Part print with two shaded views. Sizes in mm from the minimum x, y, z corner. Give positions to 0.01 mm unless a question says otherwise; leave off trailing zeros. Write each loop counter-clockwise with the first axis right and the second up, starting at its lowest first coordinate (ties: lowest second). Pieces come first, ordered by that corner, then holes.
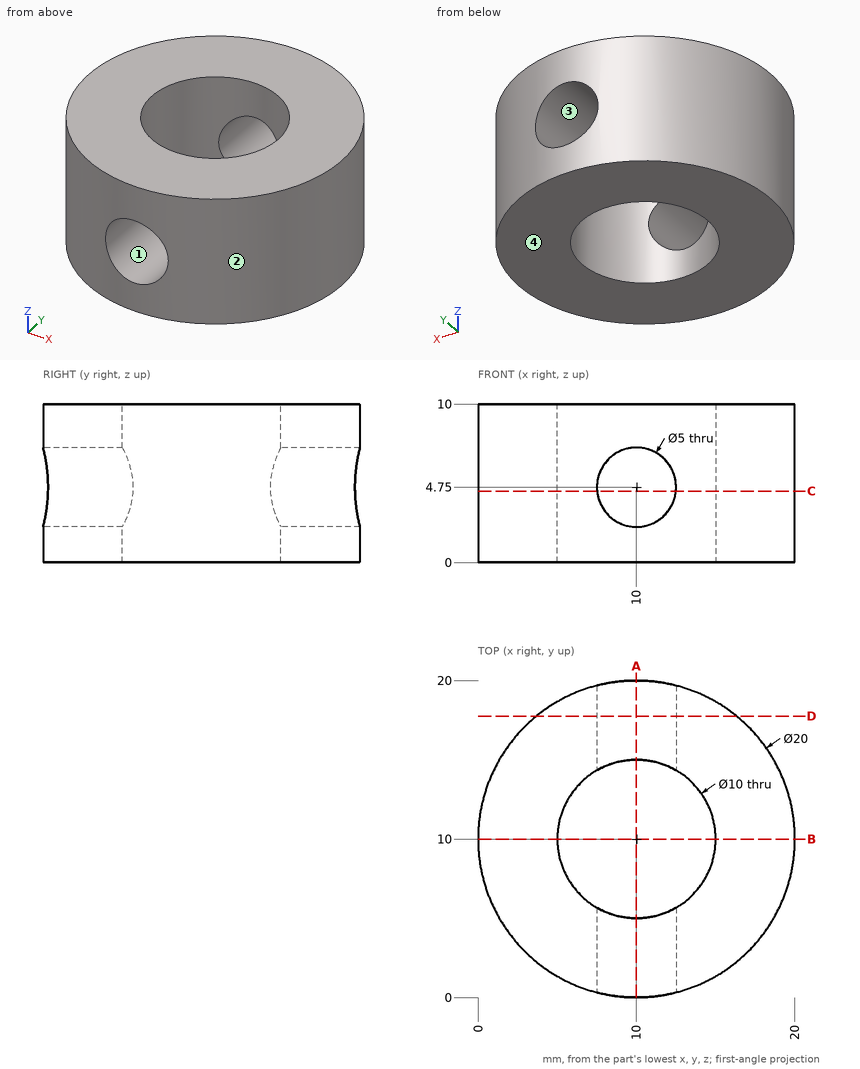
1) Flat gauge pins, fed straight in: P1, Ø2, axis at x = 7.5, z = 8.5, coming from the +Y side; P2, Ø2, axis at x = 14, z = 2, coming from the +Y side; P3, Ø1, axis at x = 3, z = 6.5, coming from the -Y side. Where does each tip first touch, or does it go through?
Check result:
P1: stops at y = 19.89
P2: stops at y = 19.54
P3: stops at y = 2.4
2) Saw through at D-D (y = 17.75). Write the cut outline in (x, z), and give its area (3 significant figures).
Check result:
outline: (3.68, 0) - (16.32, 0) - (16.32, 10) - (3.68, 10) - close; hole circle Ø5 at (10, 4.75)
area: 107 mm2
3) Saw through at C-C (z = 4.5). Write the cut outline in (x, y), and give its area (3 significant figures).
Check result:
outline: (7.51, 0.31) - (7.51, 5.66) arc R5 cw to (7.51, 14.34) - (7.51, 19.69) arc R10 ccw to start; (12.49, 0.31) arc R10 ccw to (12.49, 19.69) - (12.49, 14.34) arc R5 cw to (12.49, 5.66) - close
area: 185 mm2
4) Drill centre lines: L1, parallel to Z at x = 10, y = 3.45; L2, parallel to Y at x = 6.5, z = 2.75; L3, parallel to X at y = 10.75, z = 9.5. Where is each one in solid material? Low to high.
Check result:
L1: z = 0 to 2.25, 7.25 to 10
L2: y = 0.63 to 6.43, 13.57 to 19.37
L3: x = 0.03 to 5.06, 14.94 to 19.97
5) Mould opens along X. For the marked faces 1, 2, 3 and 4 say: +X half, -X half, draft (parallel to the pull), parting line (faces both ways), or undercut.
Check result:
face 1: undercut
face 2: parting line
face 3: undercut
face 4: draft
6) Saw through at B-B (y = 10). Write the cut outline in (x, z).
Check result:
outline: (0, 0) - (5, 0) - (5, 10) - (0, 10) - close; (15, 0) - (20, 0) - (20, 10) - (15, 10) - close
7) Saw through at A-A (x = 10). Write the cut outline in (y, z), and give its area (3 significant figures).
Check result:
outline: (0, 0) - (5, 0) - (5, 2.25) - (0, 2.25) - close; (0, 7.25) - (5, 7.25) - (5, 10) - (0, 10) - close; (15, 0) - (20, 0) - (20, 2.25) - (15, 2.25) - close; (15, 7.25) - (20, 7.25) - (20, 10) - (15, 10) - close
area: 50.0 mm2
